from build123d import *

# Parameters (mm, degrees)
SKETCH2_W           = 25
SKETCH2_H           = 20
BOSS_EXTRUDE1_DEPTH = 3
SKETCH3_R           = 3.4
SKETCH3_R_2         = 1.6
BOSS_EXTRUDE2_DEPTH = 8
LPATTERN1_COUNT     = 2
LPATTERN1_PITCH     = 17


with BuildPart() as part:
    # Sketch2 → Boss-Extrude1 (new body)
    with BuildSketch(Plane(origin=(0, 0, 0), x_dir=(0, 1, 0), z_dir=(0, 0, 1))):
        Rectangle(SKETCH2_W, SKETCH2_H)
    extrude(amount=BOSS_EXTRUDE1_DEPTH)

    # Sketch3 → Boss-Extrude2 (add)
    with BuildSketch(Plane(origin=(22.5, 12.5, 0), x_dir=(-1, 0, 0), z_dir=(0, 1, 0))):
        with Locations((34.1, 3)):
            Circle(SKETCH3_R)
        with Locations(Location((34.1, 3, 0), (0, 0, 90))):
            Circle(SKETCH3_R_2, mode=Mode.SUBTRACT)
    boss_extrude2 = extrude(amount=-BOSS_EXTRUDE2_DEPTH)

    # LPattern1: Boss-Extrude2 ×2
    with Locations(*[(0, -i * LPATTERN1_PITCH, 0) for i in range(1, LPATTERN1_COUNT)]):
        add(boss_extrude2)


solid = part.part
Source: CAD feature listing. Evaluate the final solid. Frame: model axes, mm. A direction names the side the tool comes from. Give positions to 0.01 mm unless a question says otherwise; leave off trailing zeros. Order: outer loops, then holes, each group sorted by start corner. A loop starts at its lowest first (then second) coordinate and runs counter-clockwise, first axis right, second up. Notation, with made-up numbers: (19, 30) -> (36, 30) arc R21 ccw to (36, 52) -> close; hole circle Ø5 at (54, 20). An arc over 180 degrees is marked (long way). Write item = value, one per line.
Q1. Set-up query: faces 4 (the face through (-13.16, -8.44, 2.65)), 5 (the face through (-12, -4.5, 5)), 6 (the face through (-10, 0, 1)). Return all of +Z, -Z, +X, -X, +Y, -Y with unobstructed straight access to the full face (end or side cutting, diameter ignored); none if empty.
Data:
face_4 = +Y, -Y
face_5 = +Z, -X
face_6 = +Z, -Z, -X
Q2. Cut plane C-C, the plane z = 5.75. Output: boundary loops of the cut face in (x, y), and give its area (3 significant figures).
Data:
outline = (-13.6, -12.5) -> (-9.6, -12.5) -> (-9.6, -4.5) -> (-13.6, -4.5) -> close; (-13.6, 4.5) -> (-9.6, 4.5) -> (-9.6, 12.5) -> (-13.6, 12.5) -> close
area = 64.0 mm^2
Q3. Cut plane D-D, the plane x = -7. Output: boundary loops of the cut face in (y, z).
Data:
outline = (-12.5, 0) -> (12.5, 0) -> (12.5, 3) -> (-12.5, 3) -> close
Q4. Cut plane A-A, the plane x = -11.6. Output: boundary loops of the cut face in (y, z), and give its area (3 significant figures).
Data:
outline = (-12.5, -0.4) -> (-4.5, -0.4) -> (-4.5, 1.4) -> (-12.5, 1.4) -> close; (-12.5, 4.6) -> (-4.5, 4.6) -> (-4.5, 6.4) -> (-12.5, 6.4) -> close; (4.5, -0.4) -> (12.5, -0.4) -> (12.5, 1.4) -> (4.5, 1.4) -> close; (4.5, 4.6) -> (12.5, 4.6) -> (12.5, 6.4) -> (4.5, 6.4) -> close
area = 57.6 mm^2
Q5. Material intervals for line 1 (Y direction, x = -10.25, z = 4.5); line 2 (Z direction, x = -11.6, y = 10.75); line 3 (Z direction, x = 4.5, y = 0.75), sorted ascending. Write a range as from..to.
Data:
line_1 = -12.5..-4.5, 4.5..12.5
line_2 = -0.4..1.4, 4.6..6.4
line_3 = 0..3
Q6. Pin query (flat end, axial travel): pin 1 (3 mm diameter, centred on y = -6, z = 5, fed in from +X); pin 2 (2.5 mm diameter, centred on y = 0.5, z = 2, fed in from -X); pin 3 (3 mm diameter, centred on x = -3, y = -5.5, fed in from +Z). Return the tip coordinate at first contact, or that it passes through.
Data:
pin_1 = -8.24
pin_2 = -10
pin_3 = 3
Q7. Cut plane B-B, the plane y = 9. Output: boundary loops of the cut face in (x, z), and give its area (3 significant figures).
Data:
outline = (-10, 0) -> (10, 0) -> (10, 3) -> (-8.2, 3) arc R3.4 ccw (long way) to start; hole circle Ø3.2 at (-11.6, 3)
area = 84.4 mm^2
Q8. Pull-direction query (Z, two-part tool) for faces 1 (the face through (0, 0, 0)), 2 (the face through (-13.16, 8.56, 2.65)), 3 (the face through (10, 0, 1)); classes: released by +Z, released by -Z, zero draft, split by the parting line, or undercut.
Data:
face_1 = released by -Z
face_2 = undercut
face_3 = zero draft
